The drawing under review shows one solid part. Ordinate dimensions are in mm from its lowest x, y, z. Round coordinates to 2 decimals unless told otherwise and drop trailing zeros. Order: outer loops, then holes, each group sorted by start corner. A loop starts at its lowest first (then second) coordinate and runs counter-clockwise, first axis right, second up. Notation, with made-up numbers: M 41.5,-20 L 53.5,-20 A24 cw 53.5,17 Z; hole C -11.5,75 d5. An arc over 180 degrees is marked long. Answer as a JSON object with one key per item and string values.
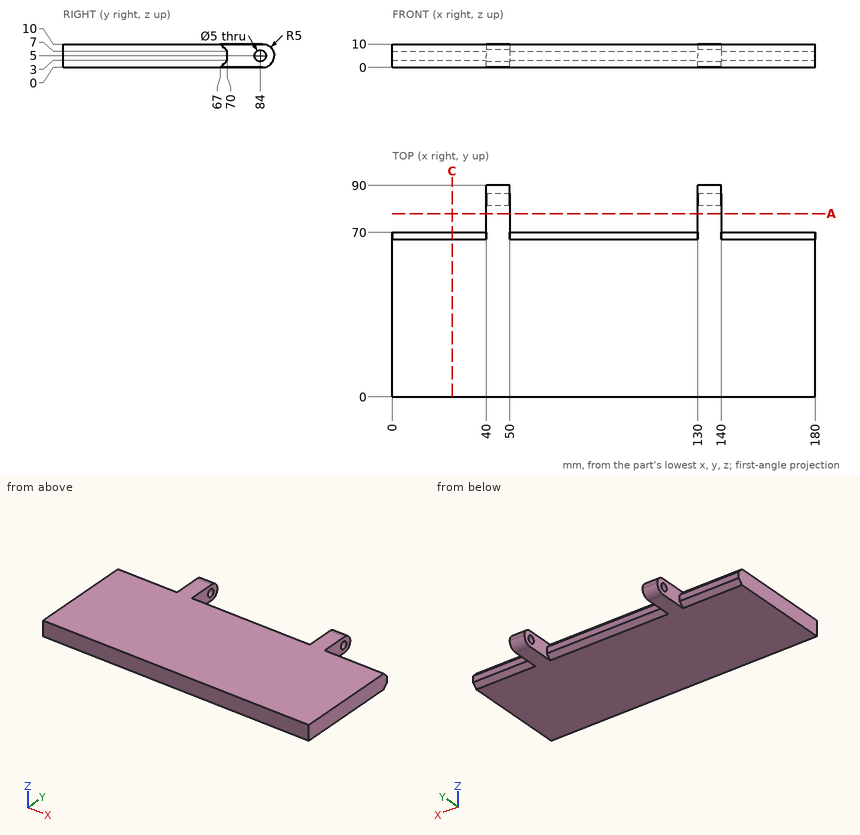
1) Insertion check: P1, Ø6, axis at y = 84, z = 5, coming from the -X side; P2, Ø5, axis at y = 79.5, z = 5.5, coming from the +X side; P3, Ø4.5, axis at x = 26.5, z = 5, coming from the +Y side. Each pin has a flat end and moves straight along its axis. Give the tip position at first contact, or say it passes through.
Geometry check:
{"P1": "stops at x = 40", "P2": "stops at x = 140", "P3": "stops at y = 70"}
2) Add section A-A on y = 78. State the section outline as (x, z) points.
Geometry check:
{"outline": "M 40,0 L 50,0 L 50,10 L 40,10 Z; M 130,0 L 140,0 L 140,10 L 130,10 Z"}
3) For L1, parallel to Z at x = 43, y = 84; L2, parallel to X at y = 77, z = 7.5; L3, parallel to Y at x = 166, z = 4.75, list the stretches that pass through material, from the lowest coordinate up.
Geometry check:
{"L1": "z = 0 to 2.5, 7.5 to 10", "L2": "x = 40 to 50, 130 to 140", "L3": "y = 0 to 70"}
4) Add section C-C on x = 25.5. State the section outline as (y, z) points.
Geometry check:
{"outline": "M 0,0 L 67,0 L 70,3 L 70,7 L 67,10 L 0,10 Z"}
